Autodesk Inventor part; units mm, degrees
ref_plane "YZ Plane" through (0, 0, 0) normal (1, 0, 0) x (0, 1, 0)
ref_plane "XZ Plane" through (0, 0, 0) normal (0, 1, 0) x (-1, 0, 0)
ref_plane "XY Plane" through (0, 0, 0) normal (0, 0, 1) x (1, 0, 0)
sketch "Sketch1" plane through (0, 0, 0) normal (0, 0, 1) x (1, 0, 0)
  circle A0 centre (0, 0) radius 1.5
  dimension "d0" = 3
extrude "Extrusion1" add sketch "Sketch1" against normal blind 30.8
fillet "Fillet1" radius 1.5 1 edges at (-1.5, 0, -30.8)
sketch "Sketch2" plane through (0, 0, 0) normal (0, 0, 1) x (1, 0, 0)
  circle A0 centre (0, 0) radius 0.7641
sketch "Sketch3" plane through (0, 0, 0) normal (0, 1, 0) x (-1, 0, 0)
  line L0 (0, 0) -> (0, 4.4513) construction
  line L1 (0, 4.4513) -> (3.2656, 6.9674) construction
  line L2 (3.2656, 6.9674) -> (6.7058, 6) construction
  line L3 (6.7058, 6) -> (9.3195, 4.0867) construction
  line L4 (9.3195, 4.0867) -> (13.4254, 1.081) construction
  spline S0 degree 4 poles (0, 0) (0, 4.4513) (3.2656, 6.9674) (6.7058, 6) (9.3195, 4.0867) (13.4254, 1.081) knots 1 1 1 1 1 2 3 3 3 3 3
  line L5 (-1.5, 0) -> (1.5, 0)
  dimension "d11" = 6
sweep "Sweep1" add profiles "Sketch2" path "Sketch3" path curves S0
sketch "Sketch4" plane through (0, 0, 0) normal (0, 0, 1) x (1, 0, 0)
  circle A0 centre (0, 0) radius 1.85
  circle A1 centre (0, 0) radius 1.5
  dimension "d8" = 3.7
extrude "Extrusion2" add sketch "Sketch4" against normal blind 10.4 draft 2 contours A0 | A1
properties part number "TempSensor_RS-762-1134"
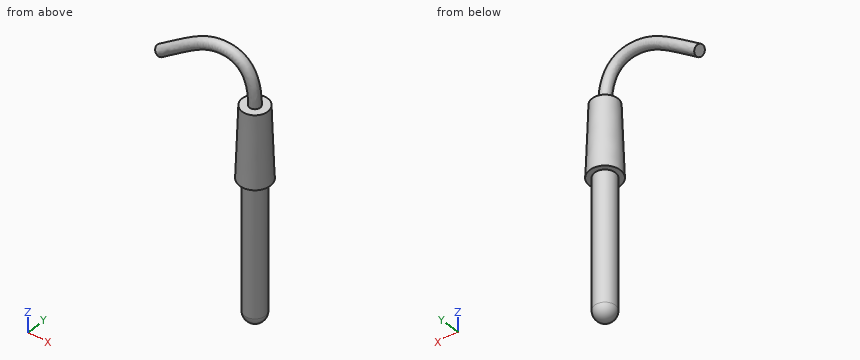
Work out the finished part from the listing and answer in its coordinate system (mm). Give positions to 0.01 mm unless a question says otherwise; leave off trailing zeros. Write each loop counter-clockwise with the first axis right and the second up, starting at its lowest first coordinate (ties: lowest second). Pieces come first, ordered by that corner, then holes. Notation, with made-up numbers: (38.5, 51) -> (73.5, 51) arc R6 ccw to (73.5, 55) -> close; hole circle Ø3 at (-9.75, 1.5). An arc over 180 degrees is marked (long way). Write item = value, one per line.
Q1. Section A-A on z = -12 is taken. Determine the outline of the cut face in (x, y), and give its area (3 significant figures).
Computed values:
outline = circle Ø3 at (0, 0)
area = 7.07 mm^2
Q2. Flat-ended cylindrical pins translate along their axes: pin 1 Ø8 at (x, z) = (-6, -25) entering from +Y; pin 2 Ø1.5 at (x, z) = (0.5, -24.5) entering from -Y; pin 3 Ø2 at (x, y) = (-12, -1) entering from -Z; pin 4 Ø1.5 at (y, z) = (-0.5, -16) entering from -X. Find the tip coordinate at first contact, or state that the pin passes through.
Computed values:
pin_1 = through
pin_2 = -1.5
pin_3 = 0.73
pin_4 = -1.5
Q3. Consider line 1 along Z through (x, y) = (1.25, -1); line 2 along X through (y, z) = (0.15, -11.5); line 3 along Z through (x, y) = (0.75, 0.85). Determine where each line is inside the solid, lowest interval first.
Computed values:
line_1 = -10.4 to 0
line_2 = -1.49 to 1.49
line_3 = -30.28 to 0
